Design review of the part shown in the three views and the two pictorial views. Dimensions are in mm from the part's minimum x, y and z. Give positions to 0.01 mm unless a question says otherwise; leave off trailing zeros. Write each loop counter-clockwise with the first axis right and the second up, starting at its lowest first coordinate (ties: lowest second). Pieces come first, ordered by that corner, then holes. Notation, with made-up numbers: (21.5, 86.25) -> (33.5, 86.25) arc R26 ccw to (33.5, 113.25) -> close; hole circle Ø10 at (-38, 15). An arc over 180 degrees is marked (long way). Use CSV: the item, a comma, the result in double quotes.
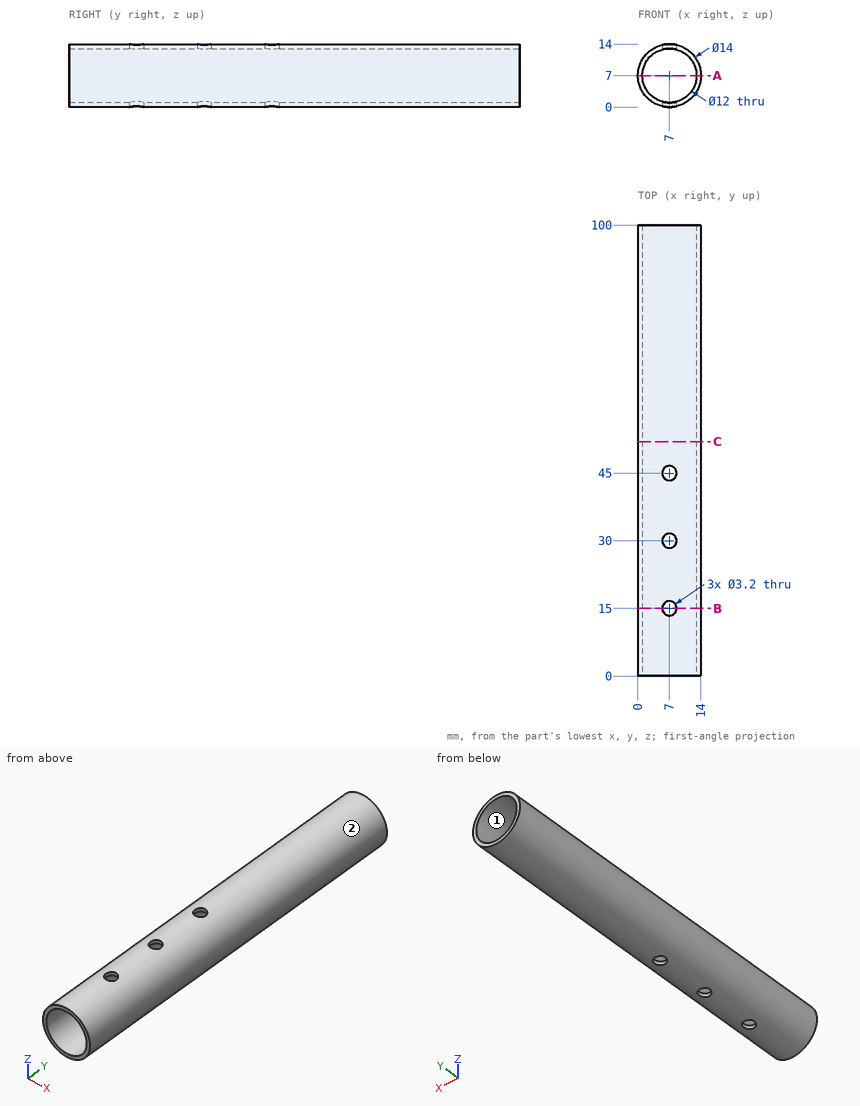
Q1. The part is to be moulded in two halves that separate along X. For the marked faces 1 and 2, say which applies: pulls with the +X half, pulls with the -X half, needs draft (parallel to the pull), parting line crosses it, or undercut.
Derived:
face 1,"undercut"
face 2,"parting line crosses it"
Q2. Consider section C-C (y = 52). Write out the cut boundary in (x, z).
Derived:
outline,"circle Ø14 at (7, 7); hole circle Ø12 at (7, 7)"
Q3. To check wall thickness, follow probe 1 along Z at (x, y) = (6.5, 83); probe 2 along Y at (x, z) = (5.75, 13); probe 3 along X at (y, z) = (84, 3.25). State the ranges of each line that lie inside material, in increasing order.
Derived:
probe 1,"z = 0.02 to 1.02, 12.98 to 13.98"
probe 2,"y = 0 to 14, 16 to 29, 31 to 44, 46 to 100"
probe 3,"x = 1.09 to 2.32, 11.68 to 12.91"
Q4. Insertion check: pin 1 (1.5 mm diameter, centred on y = 77, z = 2, fed in from -X); pin 2 (1 mm diameter, centred on y = 83.5, z = 9.5, fed in from +X); pin 3 (1.5 mm diameter, centred on x = 2, y = 54, fed in from -Z). Each pin has a flat end and moves straight along its axis. Give the tip position at first contact, or say it passes through.
Derived:
pin 1,"stops at x = 1.44"
pin 2,"stops at x = 13.71"
pin 3,"stops at z = 1.44"
Q5. Consider section A-A (z = 7). Write out the cut boundary in (x, y).
Derived:
outline,"(0, 0) -> (1, 0) -> (1, 100) -> (0, 100) -> close; (13, 0) -> (14, 0) -> (14, 100) -> (13, 100) -> close"
Q6. Consider section B-B (y = 15). Write out the cut boundary in (x, z), then the cut area to 3 significant figures.
Derived:
outline,"(5.4, 0.19) -> (5.4, 1.22) arc R6 cw to (5.4, 12.78) -> (5.4, 13.81) arc R7 ccw to start; (8.6, 0.19) arc R7 ccw to (8.6, 13.81) -> (8.6, 12.78) arc R6 cw to (8.6, 1.22) -> close"
area,"34.4 mm2"
